Geometry check sheet. Reference: the model listing, model coordinates, mm. Face numbers are marked on the shaded views. A direction names the side the tool comes from. Give positions to 0.01 mm unless a question says otherwise; leave off trailing zeros. Write each loop counter-clockwise with the first axis right and the second up, starting at its lowest first coordinate (ties: lowest second). Pieces come first, ordered by that corner, then holes. Notation, with made-up numbers: (36.5, 79) - (51.5, 79) arc R27 ccw to (51.5, 115) - close; hole circle Ø2 at (75.25, 34). An arc over 180 degrees is marked (long way). Use a Markdown table: item, result.
```python
from build123d import *

# Parameters (mm, degrees)
SKETCH2_R           = 2.45
BOSS_EXTRUDE1_DEPTH = 40
SKETCH3_W           = 20
SKETCH3_H           = 3.5
BOSS_EXTRUDE2_DEPTH = 10
SKETCH4_W           = 2
SKETCH4_H           = 3.5
CUT_EXTRUDE1_DEPTH  = 4
BOSS_EXTRUDE3_START = -1.75
BOSS_EXTRUDE3_DEPTH = 3.5


with BuildPart() as part:
    # Sketch2 → Boss-Extrude1 (new body)
    with BuildSketch(Plane.XY):
        Circle(SKETCH2_R)
    extrude(amount=BOSS_EXTRUDE1_DEPTH)

    # Sketch3 → Boss-Extrude2 (add)
    with BuildSketch(Plane(origin=(0, 0, 0), x_dir=(-1, 0, 0), z_dir=(0, 0, -1))):
        Rectangle(SKETCH3_W, SKETCH3_H)
    extrude(amount=-BOSS_EXTRUDE2_DEPTH)

    # Sketch4 → Cut-Extrude1 (cut)
    with BuildSketch(Plane(origin=(0, 0, 0), x_dir=(-1, 0, 0), z_dir=(0, 0, -1))):
        with Locations((-6.5, 0)):
            Rectangle(SKETCH4_W, SKETCH4_H)
        with Locations((6.5, 0)):
            Rectangle(SKETCH4_W, SKETCH4_H)
    extrude(amount=-CUT_EXTRUDE1_DEPTH, mode=Mode.SUBTRACT)

    # Sketch5 → Boss-Extrude3 (add)
    with BuildSketch(Plane(origin=(0, 0, 0), x_dir=(1, 0, 0), z_dir=(0, 1, 0)).offset(BOSS_EXTRUDE3_START)):
        Polygon((-1.71464282, 0), (-0.45349465, 1.109249464), (0.45349465, 1.109249464), (1.71464282, 0), (5.5, 0), (1.964975284, 3.109249464), (-1.964975284, 3.109249464), (-5.5, 0), align=None)
    extrude(amount=BOSS_EXTRUDE3_DEPTH)


solid = part.part
```
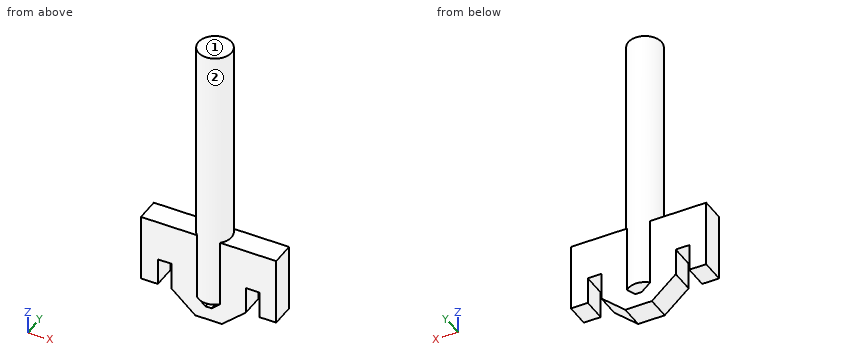
1) Section check A-A on z = 3. Record the boundary of the cut face in (x, y).
Working result:
| item | result |
|---|---|
| outline | (-10, -1.75) - (-7.5, -1.75) - (-7.5, 1.75) - (-10, 1.75) - close; (-5.5, -1.75) - (-1.71, -1.75) arc R2.45 ccw to (1.71, -1.75) - (5.5, -1.75) - (5.5, 1.75) - (1.71, 1.75) arc R2.45 ccw to (-1.71, 1.75) - (-5.5, 1.75) - close; (7.5, -1.75) - (10, -1.75) - (10, 1.75) - (7.5, 1.75) - close |
2) Material ranges on L1, parallel to Y at x = 4.75, z = 8; L2, parallel to Z at x = -0.5, y = 1.95, recorded low to high. Write a range as from..to.
Working result:
| item | result |
|---|---|
| L1 | y = -1.75..1.75 |
| L2 | z = 0..40 |
3) Section check D-D on z = 24.5. Record the boundary of the cut face in (x, y), then the cut area to 3 significant figures.
Working result:
| item | result |
|---|---|
| outline | circle Ø4.9 at (0, 0) |
| area | 18.9 mm² |
4) Section check B-B on x = 0. Record the boundary of the cut face in (y, z).
Working result:
| item | result |
|---|---|
| outline | (-2.45, 0) - (2.45, 0) - (2.45, 40) - (-2.45, 40) - close; (-1.75, -3.11) - (1.75, -3.11) - (1.75, -1.11) - (-1.75, -1.11) - close |
5) Set-up check for the marked faces 1 and 2: record each of +Z, -Z, +X, -X, +Y, -Y from which the full face is reachable in a straight line by a thin tool's end or side.
Working result:
| item | result |
|---|---|
| face 1 | +Z, +X, -X, +Y, -Y |
| face 2 | +Z |
6) Section check C-C on y = 0. Record the boundary of the cut face in (x, z).
Working result:
| item | result |
|---|---|
| outline | (-10, 0) - (-7.5, 0) - (-7.5, 4) - (-5.5, 4) - (-5.5, 0) - (-1.96, -3.11) - (1.96, -3.11) - (5.5, 0) - (5.5, 4) - (7.5, 4) - (7.5, 0) - (10, 0) - (10, 10) - (2.45, 10) - (2.45, 40) - (-2.45, 40) - (-2.45, 10) - (-10, 10) - close; hole (-1.71, 0) - (-0.45, -1.11) - (0.45, -1.11) - (1.71, 0) - close |
7) Depth check by flat-ended pin: P1, Ø1.2, axis at x = 8, y = 0, coming from the -Z side; P2, Ø2, axis at x = 6, y = -1, coming from the -Z side; P3, Ø4, axis at x = 5.5, z = 24, coming from the -Y side; P4, Ø1.1, axis at x = 5.5, y = -0.5, coming from the +Z side. Enter the tip coordinate at first touch or a pass-through.
Working result:
| item | result |
|---|---|
| P1 | stops at z = 0 |
| P2 | stops at z = -0.44 |
| P3 | passes through |
| P4 | stops at z = 10 |
